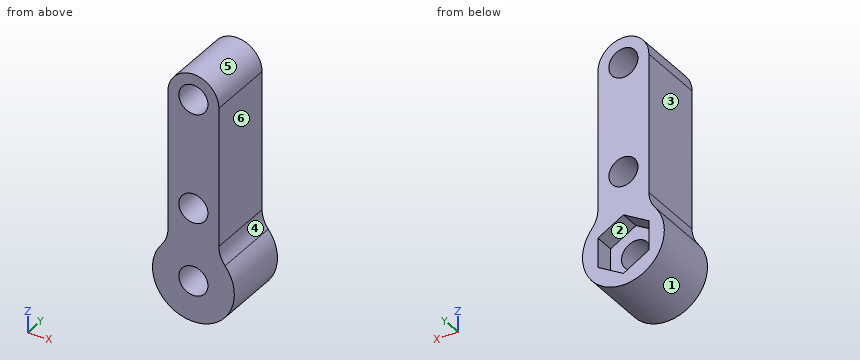
from build123d import *

# Parameters (mm, degrees)
SKETCH1_R           = 1.6
BOSS_EXTRUDE1_DEPTH = 7.5
CUT_EXTRUDE1_DEPTH  = 2.2
FILLET1_R           = 3


with BuildPart() as part:
    # Sketch1 → Boss-Extrude1 (new body)
    with BuildSketch(Plane(origin=(0, 0, 0), x_dir=(1, 0, 0), z_dir=(0, 1, 0))):
        with BuildLine():
            Line((-2.8, 0), (-2.8, 16.477217009))
            ThreePointArc((-2.8, 16.477217009), (0, 24.5), (2.8, 16.477217009))
            Line((2.8, 16.477217009), (2.8, 0))
            ThreePointArc((2.8, 0), (0, -2.8), (-2.8, 0))
        make_face()
        Circle(SKETCH1_R, mode=Mode.SUBTRACT)
        with Locations((0, 12)):
            Circle(SKETCH1_R, mode=Mode.SUBTRACT)
        with Locations((0, 20)):
            Circle(SKETCH1_R, mode=Mode.SUBTRACT)
    extrude(amount=BOSS_EXTRUDE1_DEPTH)

    # Sketch2 → Cut-Extrude1 (cut)
    with BuildSketch(Plane(origin=(0, 7.5, 0), x_dir=(1, 0, 0), z_dir=(0, 1, 0))):
        Polygon((0, 23.233161507), (-2.8, 21.616580754), (-2.8, 18.383419246), (0, 16.766838493), (2.8, 18.383419246), (2.8, 21.616580754), align=None)
    extrude(amount=-CUT_EXTRUDE1_DEPTH, mode=Mode.SUBTRACT)

    # Fillet1
    fillet1_edges = [part.edges().sort_by_distance(p)[0] for p in [
        (-2.8, 3.75, -16.477217009),
        (2.8, 3.75, -16.477217009),
    ]]
    fillet(fillet1_edges, radius=FILLET1_R)


solid = part.part
Geometry check sheet. Reference: the model listing, model coordinates, mm. Face numbers are marked on the shaded views. A direction names the side the tool comes from. Coordinates: 2 decimals unless noted, no trailing zeros. Order: outer loops, then holes, each group sorted by start corner. A loop starts at its lowest first (then second) coordinate and runs counter-clockwise, first axis right, second up. Notation, with made-up numbers: (55.5, 6.25) - (106.5, 6.25) arc R13 cw to (106.5, 20.25) - close; hole circle Ø11 at (32, 83). An arc over 180 degrees is marked (long way). Answer in a Markdown table with one row per item. Add a question column.
1) Release check for a two-part mould opening along Z. For the marked faces 1, 2, 3 and 4 record: +Z half, -Z half, draft (parallel to the pull), parting line (faces both ways), or undercut.
2) Cross-section at B-B, the plane y = 3. Record the cut outline in (x, z) (3 decimals), then the cut area to 3 significant figures.
3) Cross-section at C-C, the plane y = 6.5. Record the cut outline in (x, z) (3 decimals), then the cut area to 3 significant figures.
4) Cross-section at A-A, the plane z = -20. Record the cut outline in (x, y).
5) Cross-section at D-D, the plane z = -12. Record the cut outline in (x, y), then the cut area to 3 significant figures.
6) Material ranges on line 1 along Z through (x, y) = (0, 3.25); line 2 along X through (y, z) = (5.25, 0); line 3 along X through (y, z) = (2.8, -20), recorded low to high. Write a range as [from, to].
7) Gauge pin test, flat ends, axial feed: P1, Ø1, axis at x = 1, y = 1.5, coming from the +Z side (3 decimals); P2, Ø1.5, axis at y = 6.5, z = -19, coming from the +X side; P3, Ø3.5, axis at x = 0, z = -20, coming from the +Y side. Record the tip position at first contact, or that the pin passes through.
8) Set-up check for the marked faces 5 and 6: record each of +Z, -Z, +X, -X, +Y, -Y from which the full face is reachable in a straight line by a thin tool's end or side.
Check result:
| question | item | result |
|---|---|---|
| 1 | face 1 | parting line |
| 1 | face 2 | undercut |
| 1 | face 3 | draft |
| 1 | face 4 | +Z half |
| 2 | outline | (-3.48, -17.147) arc R4.5 ccw (long way) to (3.48, -17.147) arc R3 cw to (2.8, -15.245) - (2.8, 0) arc R2.8 ccw to (-2.8, 0) - (-2.8, -15.245) arc R3 cw to start; hole circle Ø3.2 at (0, -20); hole circle Ø3.2 at (0, -12); hole circle Ø3.2 at (0, 0) |
| 2 | area | 141 mm² |
| 3 | outline | (-3.48, -17.147) arc R4.5 ccw (long way) to (3.48, -17.147) arc R3 cw to (2.8, -15.245) - (2.8, 0) arc R2.8 ccw to (-2.8, 0) - (-2.8, -15.245) arc R3 cw to start; hole (-2.8, -21.617) - (0, -23.233) - (2.8, -21.617) - (2.8, -18.383) - (0, -16.767) - (-2.8, -18.383) - close; hole circle Ø3.2 at (0, -12); hole circle Ø3.2 at (0, 0) |
| 3 | area | 122 mm² |
| 4 | outline | (-4.5, 0) - (-1.6, 0) - (-1.6, 5.3) - (-2.8, 5.3) - (-2.8, 7.5) - (-4.5, 7.5) - close; (1.6, 0) - (4.5, 0) - (4.5, 7.5) - (2.8, 7.5) - (2.8, 5.3) - (1.6, 5.3) - close |
| 5 | outline | (-2.8, 0) - (-1.6, 0) - (-1.6, 7.5) - (-2.8, 7.5) - close; (1.6, 0) - (2.8, 0) - (2.8, 7.5) - (1.6, 7.5) - close |
| 5 | area | 18.0 mm² |
| 6 | line 1 | z = [-24.5, -21.6], [-18.4, -13.6], [-10.4, -1.6], [1.6, 2.8] |
| 6 | line 2 | x = [-2.8, -1.6], [1.6, 2.8] |
| 6 | line 3 | x = [-4.5, -1.6], [1.6, 4.5] |
| 7 | P1 | stops at z = 2.755 |
| 7 | P2 | stops at x = 4.49 |
| 7 | P3 | stops at y = 5.3 |
| 8 | face 5 | +Z, +Y, -Y |
| 8 | face 6 | +Z, +X, +Y, -Y |
